Read the model definition and answer for the solid it produces. Units are mm, in the model's axes. Face numbers are marked on the shaded views. A direction names the side the tool comes from. Give positions to 0.01 mm unless a question says otherwise; leave off trailing zeros. Order: outer loops, then holes, each group sorted by start corner. A loop starts at its lowest first (then second) coordinate and runs counter-clockwise, first axis right, second up. Notation, with made-up numbers: (43, 78.25) - (86, 78.25) arc R18 ccw to (86, 97.25) - close; hole circle Ø9 at (82, 36). An arc over 180 degrees is marked (long way). Use a Markdown table: item, result. Add a question column.
1. A cutting plane is placed at A-A on z = 8. Determine the outline of the cut face in (x, y).
2. For a pull along X with two mould halves and no side action, classify the marked faces 4, 5 and 6 as released by +X, released by -X, zero draft, split by the parting line, or undercut.
3. A cutting plane is placed at C-C on y = -3.5. Determine the outline of the cut face in (x, z) (3 decimals).
4. A cutting plane is placed at D-D on z = 24.5. State how many separate pieces and enclosed holes the cut face has, and give its area (3 significant figures).
5. Flat-ended cylindrical pins translate along their axes: P1, Ø0.9, axis at x = 19.5, y = -6.5, coming from the -Z side (3 decimals); P2, Ø1.5, axis at x = 8, y = -18.5, coming from the +Z side (3 decimals); P3, Ø21.5, axis at x = 12, z = 14, coming from the -Y side (3 decimals). Find the tip coordinate at first contact, or state that the pin passes through.
6. Which of the six approach directions +Z, -Z, +X, -X, +Y, -Y give full straight-line access (tool end or side, diameter ignored) to the marked faces 1, 2 and 3?
7. Consider L1, parallel to X at y = -32, z = 18; L2, parallel to X at y = -20.5, z = 18.5; L3, parallel to Y at x = 31.5, z = 22. Determine where each line is inside the solid, lowest interval first.
```python
from build123d import *

# Parameters (mm, degrees)
F0_W     = 38.1
F0_H     = 38.1
F1_DEPTH = 38.1
F5_DEPTH = 38.1
F7_DEPTH = 38.1
F8_W     = 25.4
F8_H     = 7.62
F9_DEPTH = 38.1


with BuildPart() as f1:
    # F0 (on Front) → F1 (new body)
    with BuildSketch(Plane.XZ):
        with Locations((19.05, 19.05)):
            Rectangle(F0_W, F0_H)
    extrude(amount=F1_DEPTH)

    # F4 (on face) → F5 (cut)
    with BuildSketch(Plane.YZ.offset(38.1)):
        Polygon((-11.43, 18.247465), (-6.35, 38.1), (-31.75, 38.1), (-26.67, 18.247465), (-21.59, 28.575), (-16.51, 28.575), align=None)
        Polygon((-6.35, 0), (0, 0), (0, 38.1), align=None)
        Polygon((-25.4, 0), (-12.7, 0), (-19.05, 15.875), align=None)
        Polygon((-38.1, 0), (-31.75, 0), (-38.1, 38.1), align=None)
    extrude(amount=-F5_DEPTH, mode=Mode.SUBTRACT)

    # F6 (on offset) → F7 (cut)
    with BuildSketch(Plane.XZ.offset(38.1)):
        Polygon((25.4, 38.1), (12.7, 38.1), (19.05, 22.225), align=None)
        Polygon((11.43, 22.225), (6.35, 0), (31.75, 0), (26.67, 22.225), (21.59, 9.525), (16.51, 9.525), align=None)
        Polygon((0, 38.1), (0, 0), (6.35, 38.1), align=None)
        Polygon((31.75, 38.1), (38.1, 0), (38.1, 38.1), align=None)
    extrude(amount=-F7_DEPTH, mode=Mode.SUBTRACT)

    # F8 (on offset) → F9 (cut)
    with BuildSketch(Plane.XY.offset(38.1)):
        with Locations((25.4, -11.43)):
            Rectangle(F8_W, F8_H)
        with Locations((12.7, -26.67)):
            Rectangle(F8_W, F8_H)
    extrude(amount=-F9_DEPTH, mode=Mode.SUBTRACT)


solid = f1.part
```
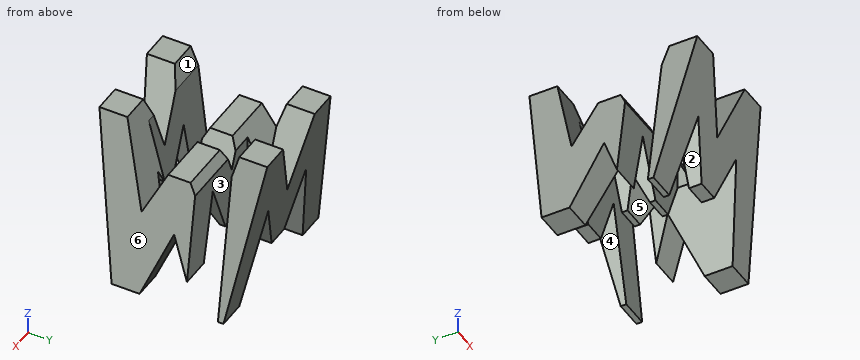
Output values:
| question | item | result |
|---|---|---|
| 1 | outline | (1.33, -33.08) - (8.18, -33.08) - (8.18, -30.48) - (1.33, -30.48) - close; (1.33, -22.86) - (8.18, -22.86) - (8.18, -22.2) - (1.33, -22.2) - close; (1.33, -15.9) - (8.18, -15.9) - (8.18, -5.02) - (1.33, -5.02) - close; (29.92, -33.08) - (36.77, -33.08) - (36.77, -22.2) - (29.92, -22.2) - close; (29.92, -15.9) - (36.77, -15.9) - (36.77, -15.24) - (29.92, -15.24) - close; (29.92, -7.62) - (36.77, -7.62) - (36.77, -5.02) - (29.92, -5.02) - close |
| 2 | face 4 | undercut |
| 2 | face 5 | zero draft |
| 2 | face 6 | released by +X |
| 3 | outline | (2.85, 17.1) - (10.259, 17.1) - (11.43, 22.225) - (13.48, 17.1) - (24.62, 17.1) - (26.67, 22.225) - (27.841, 17.1) - (35.25, 17.1) - (31.75, 38.1) - (25.4, 38.1) - (19.05, 22.225) - (12.7, 38.1) - (6.35, 38.1) - close |
| 4 | separate pieces | 6 |
| 4 | enclosed holes | 0 |
| 4 | area | 566 mm² |
| 5 | P1 | z = 9.525 |
| 5 | P2 | z = 28.575 |
| 5 | P3 | y = -35.875 |
| 6 | face 1 | +Z, +X, -X |
| 6 | face 2 | -Z, +Y, -Y |
| 6 | face 3 | +Z, -Z, +X |
| 7 | L1 | 3 to 10.46, 13.12 to 24.98, 27.64 to 35.1 |
| 7 | L2 | 3.08 to 10.58, 12.92 to 25.18, 27.52 to 35.02 |
| 7 | L3 | -35.42 to -27.63, -24.82 to -15.24, -7.62 to -2.68 |
